```python
from build123d import *

# Parameters (mm, degrees)
EXTRUDE_1_DEPTH = 2.5
M12X1_252_D     = 10.8


with BuildPart() as part:
    # Эскиз1 → Бобышка-Вытянуть1 (new body)
    with BuildSketch(Plane(origin=(0, 0, 0), x_dir=(1, 0, 0), z_dir=(0, 1, 0))):
        Polygon((0, -8.082903769), (7, -4.041451884), (7, 4.041451884), (0, 8.082903769), (-7, 4.041451884), (-7, -4.041451884), align=None)
    extrude(amount=EXTRUDE_1_DEPTH)

    # Эскиз2 → Вырез-Повернуть1 (revolve, cut)
    with BuildSketch(Plane(origin=(0, 0, 0), x_dir=(0, 0, -1), z_dir=(1, 0, 0))):
        with BuildLine():
            Line((-8.082903769, 2.5), (-8.082903769, 2))
            ThreePointArc((-8.082903769, 2), (-7.071037827, 2.373249344), (-6, 2.5))
            Line((-6, 2.5), (-8.082903769, 2.5))
        make_face()
    revolve(axis=Axis((0, 0, 0), (0, 1, 0)), mode=Mode.SUBTRACT)

    # Отверстие обработанное метчиком M12x1.252 (through all)
    with Locations(Plane.ZX.offset(2.5)):
        with Locations((0, 0)):
            Hole(M12X1_252_D / 2)


solid = part.part
```
Geometry check sheet. Reference: the model listing, model coordinates, mm. Round coordinates to 2 decimals unless told otherwise and drop trailing zeros. Order: outer loops, then holes, each group sorted by start corner. A loop starts at its lowest first (then second) coordinate and runs counter-clockwise, first axis right, second up. Notation, with made-up numbers: (47.5, -39) - (80.5, -39) arc R18 cw to (80.5, -11) - close; hole circle Ø3 at (-1, -25). An arc over 180 degrees is marked (long way). Use a Markdown table: item, result. Add a question column.
1) Thickness scan on line 1 along X through (y, z) = (1.8, 0); line 2 along Z through (x, y) = (3.5, 1.35); line 3 along Y through (x, z) = (1.25, -6). Record the ranges inside material, lowest first.
2) Section check B-B (y = 1.5). Record the cut outline in (x, z).
3) Section check A-A (z = 0). Record the cut outline in (x, y), then the cut area to 3 significant figures.
4) Mould release check, pull along Z, two halves, no side actions. Record for faces 1 (the flat face through (7, 1, 0)), 2 (the flat face through (3.45, 1.18, 6.09)), 3 (the flat face through (3.549, 1.178, -6.034)), 4 (the cylindrical face through (-5.27, 1.23, 1.17)): released by +Z, released by -Z, zero draft, split by the parting line, or undercut.
Established:
| question | item | result |
|---|---|---|
| 1 | line 1 | -7 to -5.4, 5.4 to 7 |
| 1 | line 2 | -6.06 to -4.11, 4.11 to 6.06 |
| 1 | line 3 | 0 to 2.5 |
| 2 | outline | (-7, -4.04) - (0, -8.08) - (7, -4.04) - (7, 4.04) - (0, 8.08) - (-7, 4.04) - close; hole circle Ø10.8 at (0, 0) |
| 3 | outline | (-7, 0) - (-5.4, 0) - (-5.4, 2.5) - (-6, 2.5) arc R4.59 ccw to (-7, 2.39) - close; (5.4, 0) - (7, 0) - (7, 2.39) arc R4.59 ccw to (6, 2.5) - (5.4, 2.5) - close |
| 3 | area | 7.93 mm2 |
| 4 | face 1 | zero draft |
| 4 | face 2 | released by +Z |
| 4 | face 3 | released by -Z |
| 4 | face 4 | undercut |
